The drawing under review shows one solid part. Ordinate dimensions are in mm from its lowest x, y, z. A direction names the side the tool comes from. Round coordinates to 2 decimals unless told otherwise and drop trailing zeros. Order: outer loops, then holes, each group sorted by start corner. A loop starts at its lowest first (then second) coordinate and runs counter-clockwise, first axis right, second up.
1) Clearance check with flat-ended pins moving along their axes: P1, Ø5, axis at y = 12.7, z = 12.7, coming from the +X side; P2, Ø9, axis at x = 12.5, z = 12.5, coming from the +Y side; P3, Ø5.5, axis at y = 16.5, z = 7, coming from the +X side; P4, Ø3, axis at x = 13, z = 16, coming from the +Y side. State where each tip first meets the part, or that it passes through.
2) Consider section A-A (x = 12.7). Give the boundary of the cut face in (y, z) (1 decimal).
3) Machinability: for the marked faces 4 and 5, which of the approach directions +Z, -Z, +X, -X, +Y, -Y give a long, thin tool a straight path to every point of the face, cutting with its end or side? Answer none if there is none.
4) Mouldability with a two-part tool opening along X and no side actions: class the marked faces 1, 2 and 3 as pulls with the +X half, pulls with the -X half, needs draft (parallel to the pull), parting line crosses it, or undercut.
5) To check wall thickness, follow L1, parallel to Z at x = 12.7, y = 3.7 (1 decimal); L2, parallel to X at y = 16.25, z = 8. State the ranges of each line that lie inside material, in increasing order.
6) Consider section C-C (z = 6.5). Give the boundary of the cut face in (x, y) (1 decimal).
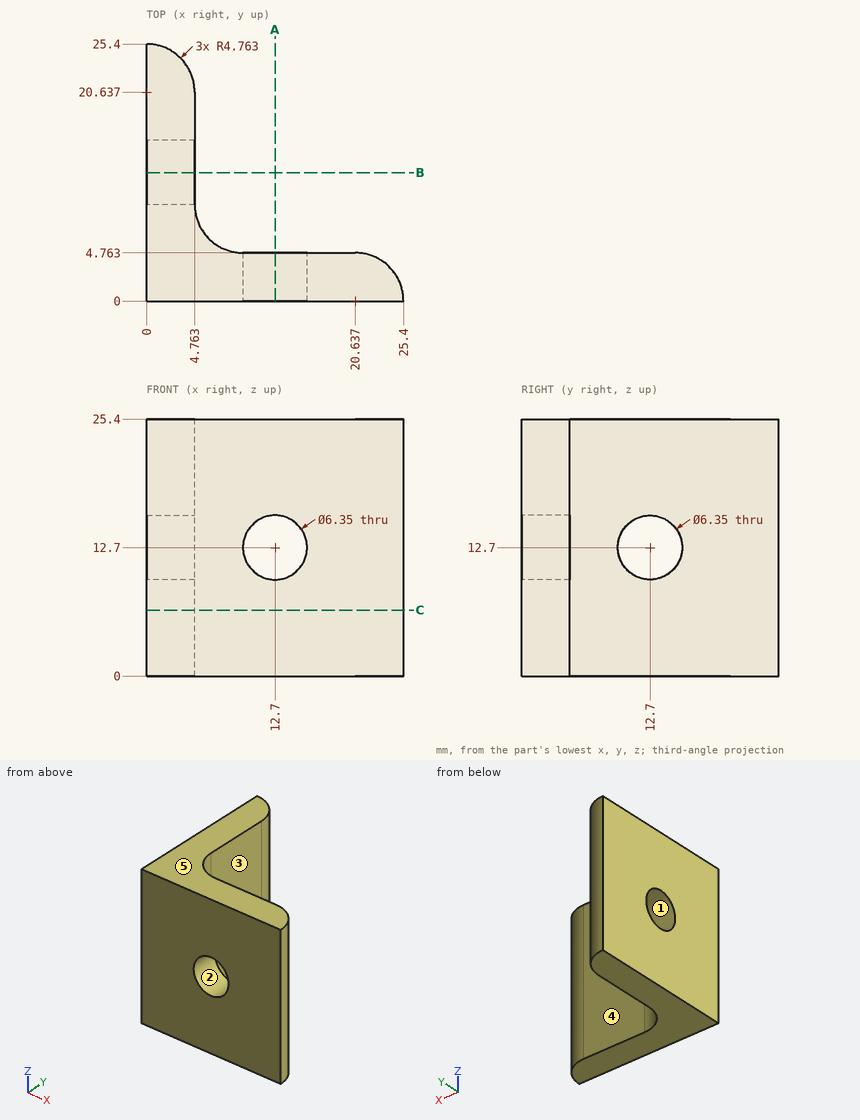
Answer below:
1. P1: passes through
1. P2: stops at y = 5.01
1. P3: stops at x = 4.76
1. P4: stops at y = 4.76
2. outline: (0, 0) - (4.8, 0) - (4.8, 9.5) - (0, 9.5) - close; (0, 15.9) - (4.8, 15.9) - (4.8, 25.4) - (0, 25.4) - close
3. face 4: +Z, -Z, +X, +Y
3. face 5: +Z, +X, -X, +Y, -Y
4. face 1: needs draft
4. face 2: undercut
4. face 3: pulls with the +X half
5. L1: z = 0 to 9.5, 15.9 to 25.4
5. L2: x = 0 to 4.76
6. outline: (0, 0) - (25.4, 0) arc R4.8 ccw to (20.6, 4.8) - (9.5, 4.8) arc R4.8 cw to (4.8, 9.5) - (4.8, 20.6) arc R4.8 ccw to (0, 25.4) - close
